Read the model definition and answer for the solid it produces. Units are mm, in the model's axes. Coordinates: 2 decimals unless noted, no trailing zeros. Write each loop counter-clockwise with the first axis right and the second up, starting at its lowest first coordinate (ties: lowest second). Pieces come first, ordered by that corner, then holes. Notation, with made-up numbers: (8, 68.5) - (32, 68.5) arc R21 cw to (32, 73.5) - close; hole circle Ø5 at (30.5, 77.5). An arc over 180 degrees is marked (long way). Return JSON: item names as keys, results as strings.
```python
from build123d import *

# Parameters (mm, degrees)
BOSS_EXTRUDE1_DEPTH = 0.8128
FILLET1_R           = 0.79375
FILLET2_R           = 1.5875


with BuildPart() as part:
    # Sketch1 → Boss-Extrude1 (new body)
    with BuildSketch(Plane.XY):
        with BuildLine():
            Line((-4.365625, 12.7), (4.365625, 12.7))
            Line((4.365625, 12.7), (4.365625, 6.629119444))
            ThreePointArc((4.365625, 6.629119444), (7.9375, 0), (4.365625, -6.629119444))
            Line((4.365625, -6.629119444), (4.365625, -12.7))
            Line((4.365625, -12.7), (-4.365625, -12.7))
            Line((-4.365625, -12.7), (-4.365625, -6.629119444))
            ThreePointArc((-4.365625, -6.629119444), (-7.9375, 0), (-4.365625, 6.629119444))
            Line((-4.365625, 6.629119444), (-4.365625, 12.7))
        make_face()
        with BuildLine():
            Line((-0.79375, -5.899971034), (-0.79375, -5.159375))
            Line((-0.79375, -5.159375), (0.79375, -5.159375))
            Line((0.79375, -5.159375), (0.79375, -5.899971034))
            ThreePointArc((0.79375, -5.899971034), (0, 5.953125), (-0.79375, -5.899971034))
        make_face(mode=Mode.SUBTRACT)
    extrude(amount=BOSS_EXTRUDE1_DEPTH)

    # Fillet1
    fillet1_edges = [part.edges().sort_by_distance(p)[0] for p in [
        (-4.365625, 12.7, 0.4064),
        (4.365625, 12.7, 0.4064),
        (4.365625, -12.7, 0.4064),
        (-4.365625, -12.7, 0.4064),
    ]]
    fillet(fillet1_edges, radius=FILLET1_R)

    # Fillet2
    fillet2_edges = [part.edges().sort_by_distance(p)[0] for p in [
        (4.365625, 6.629119444, 0.4064),
        (4.365625, -6.629119444, 0.4064),
        (-4.365625, -6.629119444, 0.4064),
        (-4.365625, 6.629119444, 0.4064),
    ]]
    fillet(fillet2_edges, radius=FILLET2_R)


solid = part.part
```
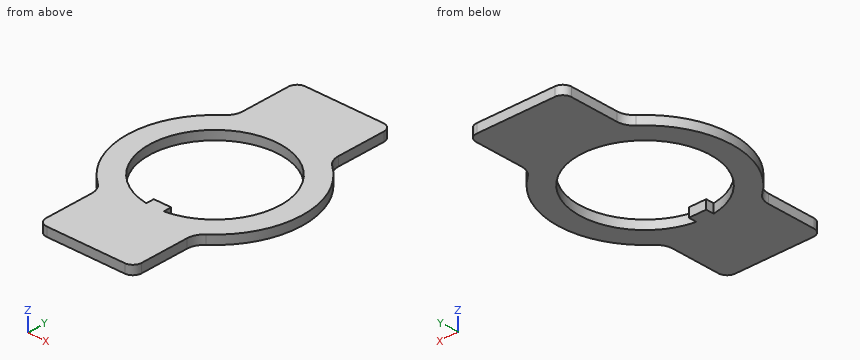
(1) A cutting plane is placed at B-B (y = 0). Determine the outline of the cut face in (x, z).
Answer:
{"outline": "(-7.94, 0) - (-5.95, 0) - (-5.95, 0.81) - (-7.94, 0.81) - close; (5.95, 0) - (7.94, 0) - (7.94, 0.81) - (5.95, 0.81) - close"}
(2) Straight lines are drawn through the part: line 1 (Y direction, x = 0, z = 0.55); line 2 (Y direction, x = -4.25, z = 0.35); line 3 (X direction, y = -3.25, z = 0.5). For each, find the intervals that lie inside material, in ascending order. Write a range as from..to.
Answer:
{"line 1": "-12.7..-5.16, 5.95..12.7", "line 2": "-12.32..-4.17, 4.17..12.32", "line 3": "-7.24..-4.99, 4.99..7.24"}
(3) A flat-ended cylindrical pin translates along its axis: P1, Ø1, axis at x = 5, y = 3, coming from the +Z side. Find the tip coordinate at first contact, or state that the pin passes through.
Answer:
{"P1": "z = 0.81"}
(4) A cutting plane is placed at A-A (x = 0). Determine the outline of the cut face in (y, z).
Answer:
{"outline": "(-12.7, 0) - (-5.16, 0) - (-5.16, 0.81) - (-12.7, 0.81) - close; (5.95, 0) - (12.7, 0) - (12.7, 0.81) - (5.95, 0.81) - close"}
(5) A cutting plane is placed at C-C (z = 0.35). Determine the outline of the cut face in (x, y) (1 decimal).
Answer:
{"outline": "(-5, -6.2) arc R1.6 cw to (-4.4, -7.4) - (-4.4, -11.9) arc R0.8 ccw to (-3.6, -12.7) - (3.6, -12.7) arc R0.8 ccw to (4.4, -11.9) - (4.4, -7.4) arc R1.6 cw to (5, -6.2) arc R7.9 ccw to (5, 6.2) arc R1.6 cw to (4.4, 7.4) - (4.4, 11.9) arc R0.8 ccw to (3.6, 12.7) - (-3.6, 12.7) arc R0.8 ccw to (-4.4, 11.9) - (-4.4, 7.4) arc R1.6 cw to (-5, 6.2) arc R7.9 ccw to start; hole (-0.8, -5.9) - (-0.8, -5.2) - (0.8, -5.2) - (0.8, -5.9) arc R6 ccw (long way) to start"}
(6) A cutting plane is placed at D-D (y = -8.5). Determine the outline of the cut face in (x, z).
Answer:
{"outline": "(-4.37, 0) - (4.37, 0) - (4.37, 0.81) - (-4.37, 0.81) - close"}
